Design review of the part built by this model. Coordinates are the model's own, in mm. A direction names the side the tool comes from. Give positions to 0.01 mm unless a question says otherwise; leave off trailing zeros. Loops run counter-clockwise (first coordinate to the right, second up) from the corner with the lowest first, then second, coordinate; pieces in that order, holes last.
from build123d import *

# Parameters (mm, degrees)
F1_DEPTH = 18
F2_R     = 3


with BuildPart() as f1:
    # F0 (on Front) → F1 (new body)
    with BuildSketch(Plane.XZ):
        with BuildLine():
            Line((57.0573561923, 212.9409522551), (0, 0))
            Line((0, 0), (35.456227742, 0))
            Line((35.456227742, 0), (111.5254217963, 163.130913087))
            ThreePointArc((111.5254217963, 163.130913087), (129.9758307308, 184.1695722906), (156.8408111482, 192))
            Line((156.8408111482, 192), (250, 192))
            Line((250, 192), (343.1591888518, 192))
            ThreePointArc((343.1591888518, 192), (370.0241692692, 184.1695722906), (388.4745782037, 163.130913087))
            Line((388.4745782037, 163.130913087), (464.543772258, 0))
            Line((464.543772258, 0), (499.2772410304, -0.1947824512))
            Line((499.2772410304, -0.1947824512), (432.8335476371, 247.7764571353))
            ThreePointArc((432.8335476371, 247.7764571353), (431.7620544452, 249.3800600209), (429.9357701582, 250))
            Line((429.9357701582, 250), (335.2377511221, 250))
            ThreePointArc((335.2377511221, 250), (333.1164307786, 249.1213203436), (332.2377511221, 247))
            Line((332.2377511221, 247), (332.2377511221, 233))
            ThreePointArc((332.2377511221, 233), (331.3590714657, 230.8786796564), (329.2377511221, 230))
            Line((329.2377511221, 230), (188.7601000309, 230))
            Line((188.7601000309, 230), (182.2377511221, 230))
            Line((182.2377511221, 230), (182.2377511221, 232.7267350544))
            Line((182.2377511221, 232.7267350544), (182.2377511221, 242.7267350544))
            Line((182.2377511221, 242.7267350544), (182.2377511221, 247))
            ThreePointArc((182.2377511221, 247), (181.3590714657, 249.1213203436), (179.2377511221, 250))
            Line((179.2377511221, 250), (178.7601000309, 250))
            Line((178.7601000309, 250), (105.3536475067, 250))
            ThreePointArc((105.3536475067, 250), (74.9155760563, 239.6676670146), (57.0573561923, 212.9409522551))
        make_face()
    extrude(amount=F1_DEPTH)

    # F2
    f2_edges = [f1.edges().sort_by_distance(p)[0] for p in [
        (28.528678, -18, 106.470476),
        (17.728114, -18, 0),
        (73.490825, -18, 81.565457),
        (129.975831, -18, 184.169572),
        (250, -18, 192),
        (370.024169, -18, 184.169572),
        (426.509175, -18, 81.565457),
        (481.910507, -18, -0.097391),
        (466.055394, -18, 123.790837),
        (431.762054, -18, 249.38006),
        (382.586761, -18, 250),
        (333.116431, -18, 249.12132),
        (332.237751, -18, 240),
        (331.359071, -18, 230.87868),
        (255.737751, -18, 230),
        (182.237751, -18, 238.5),
        (181.359071, -18, 249.12132),
        (142.295699, -18, 250),
        (74.915576, -18, 239.667667),
        (28.528678, 0, 106.470476),
        (17.728114, 0, 0),
        (73.490825, 0, 81.565457),
        (129.975831, 0, 184.169572),
        (250, 0, 192),
        (370.024169, 0, 184.169572),
        (426.509175, 0, 81.565457),
        (481.910507, 0, -0.097391),
        (466.055394, 0, 123.790837),
        (431.762054, 0, 249.38006),
        (382.586761, 0, 250),
        (333.116431, 0, 249.12132),
        (332.237751, 0, 240),
        (331.359071, 0, 230.87868),
        (255.737751, 0, 230),
        (182.237751, 0, 238.5),
        (181.359071, 0, 249.12132),
        (142.295699, 0, 250),
        (74.915576, 0, 239.667667),
        (182.237751, -9, 230),
    ]]
    fillet(f2_edges, radius=F2_R)


solid = f1.part
Q1. Tool access review of faces 4 (the face through (427.82, -0.9, 80.79)), 5 (the face through (427.82, -17.1, 80.79)), 6 (the face through (369.69, -8.92, 184.38)), 7 (the face through (332.238, -9, 240)): name each direction out of +Z, -Z, +X, -X, +Y, -Y from which nothing blocks a thin tool from reaching the whole face with its end or side.
Results:
face 4: -Z, +Y
face 5: -Z, -Y
face 6: -Z, +Y, -Y
face 7: +Z, +Y, -Y
Q2. Take a section at B-B (x = 322). Give the boundary of the cut face in (y, z).
Results:
outline: (-18, 195) arc R3 ccw to (-15, 192) - (-3, 192) arc R3 ccw to (0, 195) - (0, 227) arc R3 ccw to (-3, 230) - (-15, 230) arc R3 ccw to (-18, 227) - close
Q3. Insertion check: pin 1 (1.5 mm diameter, centred on x = 308.5, y = -14.5, fed in from +Z); pin 2 (9.5 mm diameter, centred on y = -8, z = 242, fed in from +X); pin 3 (6 mm diameter, centred on x = 11.5, y = -11.5, fed in from -Z). Each pin has a flat end and moves straight along its axis. Give the tip position at first contact, or say it passes through.
Results:
pin 1: stops at z = 230
pin 2: stops at x = 435.65
pin 3: stops at z = 0
Q4. Wall thickness on line 1 (Z direction, x = 164, y = -5.5); line 2 (X direction, y = -14.75, z = 117.5); line 3 (X direction, y = -11.25, z = 108): over which ranges is each line inside the solid? List them lowest first.
Results:
line 1: z = 192 to 250
line 2: x = 31.48 to 90.25, 409.75 to 467.74
line 3: x = 28.94 to 85.82, 414.18 to 470.29
Q5. Draft analysis for pull direction X (two halves, no side actions). For faces 1 (the face through (28.928, -8.916, 107.961)), 2 (the face through (17, -9, 0)), 3 (the face through (73.248, -17.098, 83.069)), state which applies: pulls with the +X half, pulls with the -X half, needs draft (parallel to the pull), parting line crosses it, or undercut.
Results:
face 1: pulls with the -X half
face 2: needs draft
face 3: undercut
Q6. Take a section at A-A (y = -8.25). Give the boundary of the cut face in (x, z).
Results:
outline: (0, 0) - (35.46, 0) - (111.53, 163.13) arc R50 cw to (156.84, 192) - (343.16, 192) arc R50 cw to (388.47, 163.13) - (464.54, 0) - (499.28, -0.19) - (432.83, 247.78) arc R3 ccw to (429.94, 250) - (335.24, 250) arc R3 ccw to (332.24, 247) - (332.24, 233) arc R3 cw to (329.24, 230) - (185.24, 230) arc R3 cw to (182.24, 233) - (182.24, 247) arc R3 ccw to (179.24, 250) - (105.35, 250) arc R50 ccw to (57.06, 212.94) - close
